from build123d import *

# Parameters (mm, degrees)
F0_W           = 95.2388942242
F0_H           = 63.8058483601
F1_DEPTH       = 25
F3_D           = 4.1
F3_CBORE_D     = 9.75
F3_CBORE_DEPTH = 5
F5_D           = 4.1
F5_CBORE_D     = 9.75
F5_CBORE_DEPTH = 5


with BuildPart() as f1:
    # F0 (on Top) → F1 (new body)
    with BuildSketch(Plane.XY):
        Rectangle(F0_W, F0_H)
    extrude(amount=F1_DEPTH)

    # F3 (through all)
    with Locations(Plane.XY.offset(25)):
        with Locations((-36.0746867955, -17.4044892192)):
            CounterBoreHole(F3_D / 2, F3_CBORE_D / 2, F3_CBORE_DEPTH)

    # F5 (through all)
    with Locations(Plane.XY.offset(25)):
        with Locations((34.78269279, 17.2065105289)):
            CounterBoreHole(F5_D / 2, F5_CBORE_D / 2, F5_CBORE_DEPTH)


solid = f1.part
Geometry: final body of the model. Coordinates: model frame, mm. A direction names the side the tool comes from. Give positions to 0.01 mm unless a question says otherwise; leave off trailing zeros. Write each loop counter-clockwise with the first axis right and the second up, starting at its lowest first coordinate (ties: lowest second). Pieces come first, ordered by that corner, then holes. Notation, with made-up numbers: (38.5, 56) -> (43.5, 56) arc R32 ccw to (43.5, 91) -> close; hole circle Ø8 at (-8.5, -39). An arc over 180 degrees is marked (long way). Answer as a JSON object with one key per item and string values.
1. Ray query, probe 1 along X at (y, z) = (-17.5, 19); probe 2 along X at (y, z) = (18.5, 16.25). Return the intervals inside material, ascending. Write a range as from..to.
Ans:
{"probe 1": "x = -47.62..-38.12, -34.03..47.62", "probe 2": "x = -47.62..33.19, 36.37..47.62"}
2. Access query for faces 5 (the flat face through (47.619, 0, 12)), 6 (the cylindrical face through (39.286, 15.339, 22.535)). Directions: +Z, -Z, +X, -X, +Y, -Y. A direction counts if a zero-diameter tool reaches every point of the face in a straight line with its end or side. Return the directions, or none.
Ans:
{"face 5": "+Z, -Z, +X, +Y, -Y", "face 6": "+Z"}
3. Mould query, pull axis Y, two halves, no side actions, for faces 1 (the cylindrical face through (36.41, 15.96, 9.86)), 2 (the flat face through (-36, -20, 20)), 3 (the flat face through (-1, 31.903, 12)), 4 (the flat face through (-1, 0, 0)). Classes: pulls with the +Y half, pulls with the -Y half, needs draft (parallel to the pull), parting line crosses it, or undercut.
Ans:
{"face 1": "undercut", "face 2": "undercut", "face 3": "pulls with the +Y half", "face 4": "needs draft"}
4. Cut plane A-A on x = 35. Output: boundary loops of the cut face in (y, z).
Ans:
{"outline": "(-31.9, 0) -> (15.17, 0) -> (15.17, 20) -> (12.34, 20) -> (12.34, 25) -> (-31.9, 25) -> close; (19.24, 0) -> (31.9, 0) -> (31.9, 25) -> (22.08, 25) -> (22.08, 20) -> (19.24, 20) -> close"}
5. Contact query for flat-ended pins moving along their axis: pin 1 (3.5 mm diameter, centred on x = -36.07, y = -17.4, fed in from +Z); pin 2 (5 mm diameter, centred on x = 33.5, y = 15.5, fed in from +Z); pin 3 (5 mm diameter, centred on x = 8.5, y = -1, fed in from -Z). Output: stop coordinate, or through.
Ans:
{"pin 1": "passes through", "pin 2": "stops at z = 20", "pin 3": "stops at z = 0"}
